```python
from build123d import *

# Parameters (mm, degrees)
BOSS_EXTRUDE1_OUTLINE_R = 1.35
BOSS_EXTRUDE1_DEPTH     = 6
FILLET2_R               = 4
SKETCH6_R               = 7.5
BOSS_EXTRUDE5_DEPTH     = 7
SKETCH7_R               = 1.85
CUT_EXTRUDE2_DEPTH      = 41.49625976
SKETCH8_R               = 2.1
CUT_EXTRUDE3_DEPTH      = 5
SKETCH10_R              = 8.7
SKETCH10_R_2            = 7.5
BOSS_EXTRUDE6_DEPTH     = 4.3


# Read off the part's stored shape, not the designer's step: Boss-Extrude1
with BuildPart() as part:
    # Boss-Extrude1 outline → Boss-Extrude1 (new body)
    with BuildSketch(Plane.XY):
        with BuildLine():
            add(Edge.make_bspline(
                [(19.759245017, 25.011508548), (17.277632704, 27.410130174), (11.065749819, 31.662666447), (3.898055626, 33.225), (0, 33.225), (-3.898055626, 33.225), (-11.065749819, 31.662666447), (-17.277632704, 27.410130174), (-19.759245017, 25.011508548)],
                knots=[5.561095323, 5.561095323, 5.561095323, 5.561095323, 5.890486225, 6.283185307, 6.283185307, 6.283185307, 6.675884389, 7.005275292, 7.005275292, 7.005275292, 7.005275292], degree=3))
            ThreePointArc((-19.759245017, 25.011508548), (-12.906795412, 0.176983829), (-20.263531469, -24.512854531))
            add(Edge.make_bspline(
                [(-20.263531469, -24.512854531), (-17.664381341, -27.142112776), (-11.289415252, -31.613914365), (0, -34.074654426), (11.289415252, -31.613914365), (17.664381341, -27.142112776), (20.263531469, -24.512854531)],
                knots=[2.396970099, 2.396970099, 2.396970099, 2.396970099, 2.748893572, 3.141592654, 3.534291735, 3.886215208, 3.886215208, 3.886215208, 3.886215208], degree=3))
            ThreePointArc((20.263531469, -24.512854531), (12.906795412, 0.176983829), (19.759245017, 25.011508548))
        make_face()
        with Locations((-12.92155431, -25.359978236)):
            Circle(BOSS_EXTRUDE1_OUTLINE_R, mode=Mode.SUBTRACT)
        with Locations((0, -29.225)):
            Circle(BOSS_EXTRUDE1_OUTLINE_R, mode=Mode.SUBTRACT)
        with Locations((12.92155431, -25.359978236)):
            Circle(BOSS_EXTRUDE1_OUTLINE_R, mode=Mode.SUBTRACT)
        with Locations((-12.92155431, 25.359978236)):
            Circle(BOSS_EXTRUDE1_OUTLINE_R, mode=Mode.SUBTRACT)
        with Locations((0, 29.225)):
            Circle(BOSS_EXTRUDE1_OUTLINE_R, mode=Mode.SUBTRACT)
        with Locations((12.92155431, 25.359978236)):
            Circle(BOSS_EXTRUDE1_OUTLINE_R, mode=Mode.SUBTRACT)
    extrude(amount=BOSS_EXTRUDE1_DEPTH)

    # Fillet2
    fillet2_edges = [part.edges().sort_by_distance(p)[0] for p in [
        (-20.263531469, -24.512854531, 3),
        (-19.759245017, 25.011508548, 3),
        (19.759245017, 25.011508548, 3),
        (20.263531469, -24.512854531, 3),
    ]]
    fillet(fillet2_edges, radius=FILLET2_R)

    # Sketch6 → Boss-Extrude5 (add)
    with BuildSketch(Plane.XY.offset(6)):
        Circle(SKETCH6_R)
    extrude(amount=BOSS_EXTRUDE5_DEPTH)

    # Sketch7 → Cut-Extrude2 (cut, through all)
    with BuildSketch(Plane(origin=(0, 0, 0), x_dir=(-1, 0, 0), z_dir=(0, 0, -1))):
        with Locations((0, 3.6)):
            Circle(SKETCH7_R)
        with Locations((0, -3.6)):
            Circle(SKETCH7_R)
    extrude(amount=-CUT_EXTRUDE2_DEPTH, mode=Mode.SUBTRACT)

    # Sketch8 → Cut-Extrude3 (cut)
    with BuildSketch(Plane(origin=(0, 0, 0), x_dir=(-1, 0, 0), z_dir=(0, 0, -1))):
        with Locations((10, 0)):
            Circle(SKETCH8_R)
        with Locations((0, -10)):
            Circle(SKETCH8_R)
        with Locations((-10, 0)):
            Circle(SKETCH8_R)
        with Locations((0, 10)):
            Circle(SKETCH8_R)
    extrude(amount=-CUT_EXTRUDE3_DEPTH, mode=Mode.SUBTRACT)

    # Sketch10 → Boss-Extrude6 (add)
    with BuildSketch(Plane.XY.offset(6)):
        with Locations(Location((0, 0, 0), (0, 0, 180))):
            Circle(SKETCH10_R)
        Circle(SKETCH10_R_2, mode=Mode.SUBTRACT)
    extrude(amount=BOSS_EXTRUDE6_DEPTH)


solid = part.part
```
Input: part model. Units: mm. Frame: model coordinates. A direction names the side the tool comes from. Coordinates: 2 decimals unless noted, no trailing zeros. Write each loop counter-clockwise with the first axis right and the second up, starting at its lowest first coordinate (ties: lowest second). Pieces come first, ordered by that corner, then holes. Notation, with made-up numbers: M 49,68 L 103,68 A14 cw 103,74 Z; hole C 69,6 d3. An arc over 180 degrees is marked long. Use one line per item in the form item = value.
Q1. Section C-C (y = 3.6). Return loops of the section in (x, z), plus the area to 3 significant figures.
Answer below:
outline = M -13,0 L -1.85,0 L -1.85,13 L -6.58,13 L -6.58,10.3 L -7.92,10.3 L -7.92,6 L -13,6 Z; M 1.85,0 L 13,0 L 13,6 L 7.92,6 L 7.92,10.3 L 6.58,10.3 L 6.58,13 L 1.85,13 Z
area = 212 mm²
Q2. Section D-D (z = 2.75). Count the separate pieces of the cut face and the enclosed holes in it, plus the area to 3 significant figures.
Answer below:
separate_pieces = 1
enclosed_holes = 12
area = 1,850 mm²
Q3. Set-up query: faces 5 (the face through (0.273, -7.918, 2.465)), 6 (the face through (-13.1, 26.7, 3)). Return all of +Z, -Z, +X, -X, +Y, -Y with unobstructed straight access to the full face (end or side cutting, diameter ignored); none if empty.
Answer below:
face_5 = -Z
face_6 = +Z, -Z
Q4. Draft query along Y for faces 1 (the face through (-12.905, 0.494, 2.958)), 2 (the face through (1.886, 8.493, 8.12)), 3 (the face through (0, -8, 10.3)), 4 (the face through (0, 10, 5)). Return one class per face: released by +Y, released by -Y, zero draft, split by the parting line, or undercut.
Answer below:
face_1 = undercut
face_2 = split by the parting line
face_3 = zero draft
face_4 = undercut
Q5. First-contact query: pin 1 (2.5 mm diameter, centred on x = 0, y = 29.225, fed in from -Z); pin 2 (4 mm diameter, centred on x = 0, y = -10, fed in from -Z); pin 3 (2 mm diameter, centred on y = -21, z = 2.5, fed in from +X); pin 4 (2 mm diameter, centred on x = 3, z = 6, fed in from +Y). Flat tips, straight axial feed; report the tip coordinate or a pass-through.
Answer below:
pin_1 = through
pin_2 = 5
pin_3 = 18.76
pin_4 = 33.15
Q6. Section B-B (z = 8.5). Return loops of the section in (x, y), plus the area to 3 significant figures.
Answer below:
outline = C 0,0 d17.4; hole C 0,-3.6 d3.7; hole C 0,3.6 d3.7
area = 216 mm²
Q7. Material intervals for probe 1 along Y at (x, z) = (0, 7.5); probe 2 along X at (y, z) = (1.5, 1.75); probe 3 along Z at (x, y) = (-11.5, 2.5), sorted ascending. Write a range as from..to.
Answer below:
probe_1 = -8.7..-5.45, -1.75..1.75, 5.45..8.7
probe_2 = -12.91..-11.47, -8.53..8.53, 11.47..12.91
probe_3 = 0..6
Q8. Section A-A (y = -3.6). Return loops of the section in (x, z), plus the area to 3 significant figures.
Answer below:
outline = M -13.1,0 L -1.85,0 L -1.85,13 L -6.58,13 L -6.58,10.3 L -7.92,10.3 L -7.92,6 L -13.1,6 Z; M 1.85,0 L 13.1,0 L 13.1,6 L 7.92,6 L 7.92,10.3 L 6.58,10.3 L 6.58,13 L 1.85,13 Z
area = 213 mm²
